Input: part model. Units: mm. Frame: model coordinates. Round coordinates to 2 decimals unless told otherwise and drop trailing zeros. Order: outer loops, then holes, each group sorted by start corner. A loop starts at its lowest first (then second) coordinate and runs counter-clockwise, first axis right, second up.
Item 1: Cut plane D-D on y = 6.25. Output: boundary loops of the cut face in (x, z).
Item 2: First-contact query: pin 1 (2 mm diameter, centred on x = 0, y = 6, fed in from +Z); pin 2 (1 mm diameter, centred on x = -1.5, z = 0, fed in from +Y). Flat tips, straight axial feed; report the tip coordinate or a pass-through.
Item 3: Cut plane C-C on y = 2.5. Output: boundary loops of the cut face in (x, z), then the cut area to 3 significant figures.
Item 4: Mould query, pull axis X, two halves, no side actions, for faces 1 (the flat face through (0.87, 0.87, 0.49)), 2 (the cylindrical face through (2, 3, 0)). Classes: released by +X, released by -X, zero draft, split by the parting line, or undercut.
Item 5: Cut plane A-A on y = 1. Output: boundary loops of the cut face in (x, z), then the cut area to 3 significant figures.
Item 6: Cut plane B-B on x = 0. Output: boundary loops of the cut face in (y, z), then the cut area to 3 significant figures.
Item 7: Line query: L1, parallel to Z at x = 0.1, y = 2.75; L2, parallel to Z at x = -1.1, y = 0.75; L3, parallel to Y at x = -0.6, z = 1.3. Output: solid intervals per line, ascending.
```python
from build123d import *

# Parameters (mm, degrees)
CHAMFER_1_SIZE      = 0.2
CUT_EXTRUDE_1_DEPTH = 1.5
CHAMFER_3_SIZE      = 0.25


with BuildPart() as part:
    # Эскиз1 → Повернуть1 (revolve)
    with BuildSketch(Plane.XY, mode=Mode.PRIVATE) as revolve_1_sk:
        with BuildLine():
            Line((0, 0), (-2, 0))
            Line((-2, 0), (-2, 4.902209534))
            Line((-2, 4.902209534), (-1.366190379, 6))
            Line((-1.366190379, 6), (-1.166190379, 6))
            ThreePointArc((-1.166190379, 6), (-0.707106781, 6.580776406), (0, 6.8))
            Line((0, 6.8), (0, 0))
        make_face()
    revolve(revolve_1_sk.sketch.rotate(Axis((0, 6.8, 0), (0, -1, 0)), 270), axis=Axis((0, 6.8, 0), (0, -1, 0)))

    # Фаска1
    chamfer_1_edges = [part.edges().sort_by_distance(p)[0] for p in [
        (0, 0, -2),
    ]]
    chamfer(chamfer_1_edges, length=CHAMFER_1_SIZE)

    # Эскиз2 → Вырез-Вытянуть1 (cut)
    with BuildSketch(Plane.XZ):
        Polygon((1.154700538, 0), (0.577350269, 1), (-0.577350269, 1), (-1.154700538, 0), (-0.577350269, -1), (0.577350269, -1), align=None)
    extrude(amount=-CUT_EXTRUDE_1_DEPTH, mode=Mode.SUBTRACT)

    # Фаска3
    chamfer_3_edges = [part.edges().sort_by_distance(p)[0] for p in [
        (0.8660254037844386, 0, -0.5000000000000002),
        (0.8660254037844386, 0, 0.5000000000000007),
        (0, 0, 1),
        (-0.8660254037844393, 0, 0.5000000000000004),
        (-0.8660254037844393, 0, -0.5000000000000003),
        (0, 0, -1),
    ]]
    chamfer(chamfer_3_edges, length=CHAMFER_3_SIZE)


solid = part.part
```
From the geometry:
1. outline: circle Ø2.07 at (0, 0)
2. pin 1: stops at z = 1.94
2. pin 2: stops at y = 6.3
3. outline: circle Ø4 at (0, 0)
3. area: 12.6 mm2
4. face 1: undercut
4. face 2: split by the parting line
5. outline: circle Ø4 at (0, 0); hole (-1.15, 0) - (-0.58, -1) - (0.58, -1) - (1.15, 0) - (0.58, 1) - (-0.58, 1) - close
5. area: 9.10 mm2
6. outline: (0, -1.8) - (0.2, -2) - (4.9, -2) - (6, -1.37) - (6, -1.17) arc R1.25 ccw to (6, 1.17) - (6, 1.37) - (4.9, 2) - (0.2, 2) - (0, 1.8) - (0, 1.25) - (0.25, 1) - (1.5, 1) - (1.5, -1) - (0.25, -1) - (0, -1.25) - close
6. area: 21.6 mm2
7. L1: z = -2 to 2
7. L2: z = -1.67 to -0.09, 0.09 to 1.67
7. L3: y = 0 to 5.89
